from build123d import *

# Parameters (mm, degrees)
BOSS_EXTRUDE1_DEPTH = 6
SKETCH2_R           = 3
SKETCH2_R_2         = 2.5
CUT_EXTRUDE1_DEPTH  = 6


with BuildPart() as part:
    # Sketch1 → Boss-Extrude1 (new body)
    with BuildSketch(Plane(origin=(0, 0, 0), x_dir=(1, 0, 0), z_dir=(0, 1, 0))):
        Polygon((418, 244), (424, 244), (424, 288), (430, 288), (430, 0), (424, 0), (424, 44), (418, 44), (418, 0), (0, 0), (0, 44), (-6, 44), (-6, 0), (-12, 0), (-12, 288), (-6, 288), (-6, 244), (0, 244), (0, 288), (418, 288), align=None)
    extrude(amount=BOSS_EXTRUDE1_DEPTH)

    # Sketch2 → Cut-Extrude1 (cut)
    with BuildSketch(Plane(origin=(0, 6, 0), x_dir=(1, 0, 0), z_dir=(0, 1, 0))):
        with Locations(Location((150, 135, 0), (0, 0, 270))):
            Circle(SKETCH2_R)
        with Locations(Location((150, 153, 0), (0, 0, 270))):
            Circle(SKETCH2_R)
        with Locations(Location((141, 144, 0), (0, 0, 270))):
            Circle(SKETCH2_R_2)
        with Locations(Location((159, 144, 0), (0, 0, 270))):
            Circle(SKETCH2_R_2)
        with BuildLine():
            add(Edge.make_bspline(
                [(250, 154), (231.978482396, 153.666282679), (221.933324248, 152.446887217), (221.5, 144)],
                knots=[0, 0, 0, 0, 1, 1, 1, 1], degree=3))
            add(Edge.make_bspline(
                [(250, 134), (231.978482396, 134.333717321), (221.933324248, 135.553112783), (221.5, 144)],
                knots=[0, 0, 0, 0, 1, 1, 1, 1], degree=3))
            add(Edge.make_bspline(
                [(250, 134), (268.021517604, 134.333717321), (278.066675752, 135.553112783), (278.5, 144)],
                knots=[0, 0, 0, 0, 1, 1, 1, 1], degree=3))
            add(Edge.make_bspline(
                [(250, 154), (268.021517604, 153.666282679), (278.066675752, 152.446887217), (278.5, 144)],
                knots=[0, 0, 0, 0, 1, 1, 1, 1], degree=3))
        make_face()
    extrude(amount=-CUT_EXTRUDE1_DEPTH, mode=Mode.SUBTRACT)


solid = part.part
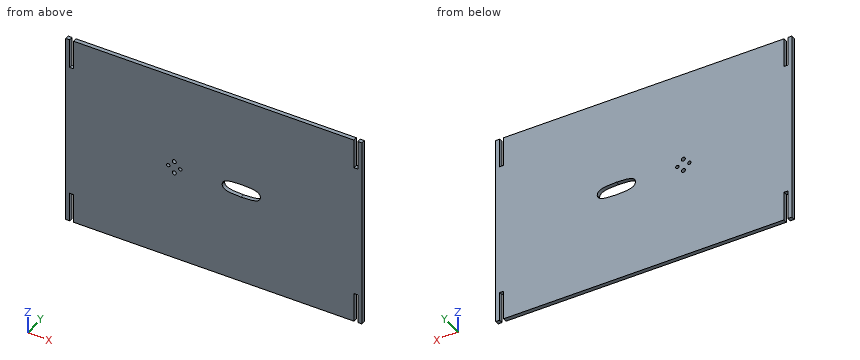
The model under review builds one solid part; all positions refer to its coordinate system, in mm. Coordinates: 2 decimals unless noted, no trailing zeros. Answer as CSV lines item,"result".
(1) Clearance check with flat-ended pins moving along their axes: pin 1 Ø4.5 at (x, z) = (141, -144) entering from -Y; pin 2 Ø1.8 at (x, y) = (-3.5, 3.5) entering from -Z. State where each tip first meets the part, or that it passes through.
Data:
pin 1,"passes through"
pin 2,"stops at z = -244"
(2) We need section A-A (y = 1.75). Count the separate pieces of the cut face and the enclosed holes in it, plus the area to 3 significant figures.
Data:
separate pieces,"1"
enclosed holes,"5"
area,"125,000 mm2"
(3) For line 1 along X through (y, z) = (2.9, -144); line 2 along X through (y, z) = (1.5, -249.5); line 3 along Z through (x, y) = (150, 4.5), list the stretches that pass through material, from the lowest coordinate up. Write a range as [from, to].
Data:
line 1,"x = [-12, 138.5], [143.5, 156.5], [161.5, 221.5], [278.5, 430]"
line 2,"x = [-12, -6], [0, 418], [424, 430]"
line 3,"z = [-288, -156], [-150, -138], [-132, 0]"
